For this review, take the finished solid that the model builds, in its own axes (mm). A direction names the side the tool comes from. Round coordinates to 2 decimals unless told otherwise and drop trailing zeros. Order: outer loops, then holes, each group sorted by start corner. A loop starts at its lowest first (then second) coordinate and runs counter-clockwise, first axis right, second up. Notation, with made-up numbers: (-39, 21.5) -> (1, 21.5) arc R28 cw to (1, 40.5) -> close; hole circle Ø8 at (34, -11.5). An arc over 180 degrees is marked (long way). Use a Markdown table: item, result. Add a question column.
1) Consider section B-B (z = 23). State the section outline as (x, y) points.
2) Wall thickness on line 1 along Y through (x, z) = (68.5, 8); line 2 along Z through (x, y) = (71, 9); line 3 along X through (y, z) = (23, 13): over which ranges is each line inside the solid? List them lowest first. Write a range as [from, to].
3) Consider section C-C (x = 68). State the section outline as (y, z) points.
4) Draft analysis for pull direction X (two halves, no side actions). For faces 4 (the face through (0, 25, 14)), 5 (the face through (55, 9, 25)), 6 (the face through (17.232, 9.22, 10.846)), state which applies: pulls with the +X half, pulls with the -X half, needs draft (parallel to the pull), parting line crosses it, or undercut.
5) Machinability: for faces 1 (the face through (32.652, 25.358, 24.958)), 2 (the face through (91, 36, 19)), 3 (the face through (80, 43, 22)), which of the approach directions +Z, -Z, +X, -X, +Y, -Y give a long, thin tool a straight path to every point of the face, cutting with its end or side? Answer none if there is none.
6) Clearance check with flat-ended pins moving along their axes: P1, Ø3, axis at x = 88.5, z = 20.5, coming from the -Y side; P2, Ø11.5, axis at x = 22.23, y = 41, coming from the +Z side; P3, Ø6.5, axis at y = 7, z = 26, coming from the +X side; P4, Ø1, axis at y = 15, z = 4.5, coming from the +X side. State where each tip first meets the part, or that it passes through.
7) Consider section A-A (y = 25). State the section outline as (x, z) points.
8) Consider section D-D (z = 7.5). State the section outline as (x, y) points, plus the area to 3 significant figures.
```python
from build123d import *

# Parameters (mm, degrees)
F0_R     = 5
F1_DEPTH = 22
F2_DEPTH = 28
F3_DEPTH = 22
F4_DEPTH = 16


with BuildPart() as f1:
    # F0 (on Top) → F1 (new body)
    with BuildSketch(Plane.XY):
        with BuildLine():
            ThreePointArc((11, 50), (7.651514, 25), (11, 0))
            Line((11, 0), (37.26803, 0))
            ThreePointArc((37.26803, 0), (32.651514, 25), (37.26803, 50))
            Line((37.26803, 50), (11, 50))
        make_face()
        with Locations((22.227637, 9)):
            Circle(F0_R, mode=Mode.SUBTRACT)
        with Locations((22.227637, 41)):
            Circle(F0_R, mode=Mode.SUBTRACT)
    extrude(amount=F1_DEPTH)

    # F0 (on Top) → F2 (join)
    with BuildSketch(Plane.XY):
        with BuildLine():
            Line((0, 50), (0, 0))
            Line((0, 0), (11, 0))
            ThreePointArc((11, 0), (7.651514, 25), (11, 50))
            Line((11, 50), (0, 50))
        make_face()
        with BuildLine():
            ThreePointArc((37.26803, 50), (32.651514, 25), (37.26803, 0))
            Line((37.26803, 0), (55, 0))
            Line((55, 0), (55, 19.042652))
            ThreePointArc((55, 19.042652), (53.7, 25), (55, 30.957348))
            Line((55, 30.957348), (55, 50))
            Line((55, 50), (37.26803, 50))
        make_face()
    extrude(amount=F2_DEPTH)

    # F0 (on Top) → F3 (join)
    with BuildSketch(Plane.XY):
        with BuildLine():
            Line((97, 50), (55, 50))
            Line((55, 50), (55, 30.957348))
            ThreePointArc((55, 30.957348), (64.823961, 38.94284), (77.137286, 36))
            Line((77.137286, 36), (105.082904, 36))
            Line((105.082904, 36), (97, 50))
        make_face()
        with BuildLine():
            Line((55, 19.042652), (55, 0))
            Line((55, 0), (97, 0))
            Line((97, 0), (105.082904, 14))
            Line((105.082904, 14), (77.137286, 14))
            ThreePointArc((77.137286, 14), (64.823961, 11.05716), (55, 19.042652))
        make_face()
    extrude(amount=F3_DEPTH)

    # F0 (on Top) → F4 (join)
    with BuildSketch(Plane.XY):
        with BuildLine():
            ThreePointArc((77.137286, 36), (82.3, 25), (77.137286, 14))
            Line((77.137286, 14), (105.082904, 14))
            Line((105.082904, 14), (108, 19.052559))
            Line((108, 19.052559), (108, 30.947441))
            Line((108, 30.947441), (105.082904, 36))
            Line((105.082904, 36), (77.137286, 36))
        make_face()
    extrude(amount=F4_DEPTH)


solid = f1.part
```
Results list:
| question | item | result |
|---|---|---|
| 1 | outline | (0, 0) -> (11, 0) arc R95 cw to (11, 50) -> (0, 50) -> close; (37.27, 0) -> (55, 0) -> (55, 19.04) arc R14.3 cw to (55, 30.96) -> (55, 50) -> (37.27, 50) arc R70 ccw to start |
| 2 | line 1 | [0, 10.71], [39.29, 50] |
| 2 | line 2 | [0, 22] |
| 2 | line 3 | [0, 53.84], [82.16, 108] |
| 3 | outline | (0, 0) -> (10.7, 0) -> (10.7, 22) -> (0, 22) -> close; (39.3, 0) -> (50, 0) -> (50, 22) -> (39.3, 22) -> close |
| 4 | face 4 | pulls with the -X half |
| 4 | face 5 | pulls with the +X half |
| 4 | face 6 | undercut |
| 5 | face 1 | +Z |
| 5 | face 2 | +Z, +X |
| 5 | face 3 | +Z, +X, +Y, -Y |
| 6 | P1 | y = 0 |
| 6 | P2 | z = 22 |
| 6 | P3 | x = 55 |
| 6 | P4 | x = 105.95 |
| 7 | outline | (0, 0) -> (53.7, 0) -> (53.7, 28) -> (32.65, 28) -> (32.65, 22) -> (7.65, 22) -> (7.65, 28) -> (0, 28) -> close; (82.3, 0) -> (108, 0) -> (108, 16) -> (82.3, 16) -> close |
| 8 | outline | (0, 0) -> (97, 0) -> (108, 19.05) -> (108, 30.95) -> (97, 50) -> (0, 50) -> close; hole circle Ø10 at (22.23, 9); hole circle Ø10 at (22.23, 41); hole (55, 19.04) arc R14.3 ccw to (77.14, 14) arc R14.3 ccw to (77.14, 36) arc R14.3 ccw to (55, 30.96) arc R14.3 ccw to start |
| 8 | area | 4,390 mm2 |
